```python
from build123d import *

# Parameters (mm, degrees)
BOSS_EXTRUDE1_DEPTH     = 12.7
FILLET2_SIZE            = 41.275
FILLET2_SIZE_2          = 69.85
FILLET3_R               = 25.4
FILLET4_R               = 19.05
FILLET6_R               = 127
CUT_EXTRUDE1_REACH      = 634.314
SKETCH3_W               = 241.600142069
SKETCH3_H               = 584.2
F_8_CLEARANCE_HOLE1_D   = 4.9149
F_1_4_CLEARANCE_HOLE1_D = 7.14248


with BuildPart() as part:
    # Sketch1 → Boss-Extrude1 (new body)
    with BuildSketch(Plane.XY):
        Polygon((-228.088766336, 0), (228.088766336, 0), (228.088766336, -443.878997916), (241.600142069, -584.2), (230.934597128, -584.2), (196.338766336, -463.55), (79.375, -463.55), (79.375, -363.22), (-79.375, -363.22), (-79.375, -463.55), (-196.338766336, -463.55), (-230.934597128, -584.2), (-241.600142069, -584.2), (-228.088766336, -443.878997916), align=None)
    extrude(amount=BOSS_EXTRUDE1_DEPTH)

    # Fillet2
    # a fillet whose section is not a circle: 69.85, 41.275 mm, written as the material it adds along each edge
    with BuildSketch(Plane(origin=(-79.375, -363.22, 0), x_dir=(1, 0, 0), z_dir=(0, 0, 1))) as fillet2_piece_1:
        with BuildLine():
            Bezier((FILLET2_SIZE, 0), (0, 0), (0, -FILLET2_SIZE_2), weights=[1, 1.5, 1])
            Line((0, -FILLET2_SIZE_2), (0, 0))
            Line((0, 0), (FILLET2_SIZE, 0))
        make_face()
    extrude(amount=12.7)

    # Fillet3
    fillet3_edges = [part.edges().sort_by_distance(p)[0] for p in [
        (-79.375, -463.55, 6.35),
    ]]
    fillet(fillet3_edges, radius=FILLET3_R)

    # Fillet4
    fillet4_edges = [part.edges().sort_by_distance(p)[0] for p in [
        (-196.338766336, -463.55, 6.35),
    ]]
    fillet(fillet4_edges, radius=FILLET4_R)

    # Fillet5
    # a fillet whose section is not a circle: 50.8, 22.225 mm, written as the material it takes off along each edge
    with BuildSketch(Plane(origin=(-230.934597128, -584.2, -116.185737858), x_dir=(0.2756373558169957, 0.9612616959383199, 0), z_dir=(0, 0, 1))) as fillet5_piece_1:
        with BuildLine():
            Bezier((46.474295143, 0), (0, 0), (-2.35779901, 8.222622324), weights=[1, 2.333333333, 1])
            Line((-2.35779901, 8.222622324), (0, 0))
            Line((0, 0), (46.474295143, 0))
        make_face()
    extrude(amount=245.071475716, mode=Mode.SUBTRACT)

    # Fillet6
    # the kernel refuses this fillet: 127 mm, written as the material it adds along each edge
    with BuildSketch(Plane(origin=(-228.088766336, -443.878997916, 0), x_dir=(0, 1, 0), z_dir=(0, 0, 1))) as fillet6_piece_1:
        with BuildLine():
            CenterArc((FILLET6_R * 0.0480334444852, FILLET6_R), FILLET6_R, 264.5, 5.5)
            Line((-FILLET6_R * 0.047812308035, FILLET6_R * 0.00460380163282), (0, 0))
            Line((0, 0), (FILLET6_R * 0.0480334444852, 0))
        make_face()
    extrude(amount=12.7)

    # Sketch3 → Cut-Extrude1 (cut, up to next)
    with BuildSketch(Plane.XY.offset(12.7), mode=Mode.PRIVATE) as cut_extrude1_sk1:
        with Locations((120.800071035, -292.1)):
            Rectangle(SKETCH3_W, SKETCH3_H)
    cut_extrude1_tool1 = extrude(cut_extrude1_sk1.sketch, amount=-CUT_EXTRUDE1_REACH, mode=Mode.PRIVATE) & part.part
    add(cut_extrude1_tool1.solids().sort_by_distance((120.800071, -292.1, 12.7))[0], mode=Mode.SUBTRACT)

    # Mirror5: part across plane


with BuildPart() as part_1:
    add(part.part)
    add(part.part.mirror(Plane(origin=(0, 0, -0.35025), x_dir=(0, 0, 1), z_dir=(-1, 0, 0))))

    # #8 Clearance Hole1 (through all)
    with Locations(Plane(origin=(0, 0, 0), x_dir=(-1, 0, 0), z_dir=(0, 0, -1))):
        with Locations((12.077216058, -342.5825), (-12.077216058, -342.5825)):
            Hole(F_8_CLEARANCE_HOLE1_D / 2)

    # 1/4 Clearance Hole1 (through all)
    with Locations(Plane(origin=(0, 0, 0), x_dir=(-1, 0, 0), z_dir=(0, 0, -1))):
        with Locations((0, -352.7425), (0, -332.4225)):
            Hole(F_1_4_CLEARANCE_HOLE1_D / 2)


solid = part_1.part
```
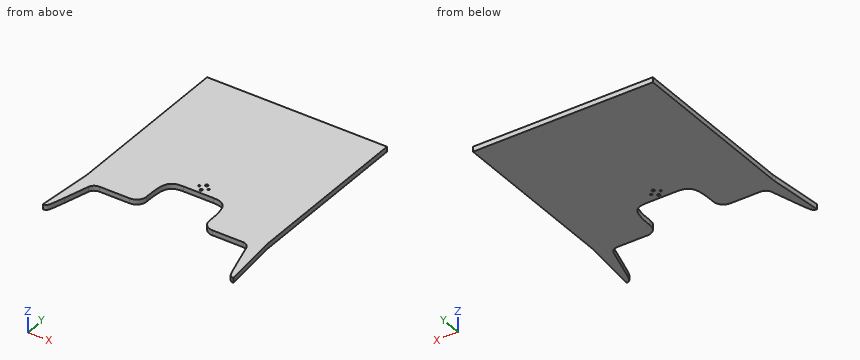
The listing builds one solid part. Answer for the finished solid, in the listing's coordinates (mm). Coordinates: 2 decimals unless noted, no trailing zeros. Loops run counter-clockwise (first coordinate to the right, second up) from the corner with the lowest first, then second, coordinate; pieces in that order, holes last. Notation, with made-up numbers: M 25,-6.5 L 71,-6.5 A36 cw 71,27.5 Z; hole C 61.5,50 d4. An arc over 180 degrees is marked long. Answer as CSV lines item,"result". Start each with the question number.
(1) The part is cut by section B-B (x = 127.5). Give the vertices of the cut face in (y, z).
(2) The part is cut by section A-A (y = -526). Give the vertices of the cut face in (x, z).
(3) The part is cut by section C-C (y = -93.5). Give the vertices of the cut face in (x, z), and give its area (3 significant figures).
(4) Given pin 1 (1.5 mm diameter, centred on y = -404, z = 8.5, fed in from +X); pin 2 (3 mm diameter, centred on y = -151, z = 7.5, fed in from -X); pin 3 (4 mm diameter, centred on x = 1.5, z = 5.5, fed in from -Y); pin 4 (3 mm diameter, centred on x = -12.08, y = -342.58, fed in from +Z), each flat-ended and moving along its own axis, determine where each tip first touches the part or whether it passes through.
(5) The part is cut by section D-D (z = 3.75). State how many separate pieces and enclosed holes the cut face has, and give its area (3 significant figures).
(6) Find the intervals of material crossed by L1, parallel to Y at x = 0, z = 9.5; L2, parallel to Y at x = -2, z = 2; L3, parallel to X at y = -343.5, z = 8, in increasing order. Write a range as [from, to].
Determined:
1,outline,"M -463.55,0 L 0,0 L 0,12.7 L -463.55,12.7 Z"
2,outline,"M -236,0 L -214.25,0 L -214.25,12.7 L -236,12.7 Z; M 214.25,0 L 236,0 L 236,12.7 L 214.25,12.7 Z"
3,outline,"M -228.09,0 L 228.09,0 L 228.09,12.7 L -228.09,12.7 Z"
3,area,"5,790 mm2"
4,pin 1,"x = 228.09"
4,pin 2,"x = -228.09"
4,pin 3,"y = -363.22"
4,pin 4,"through"
5,separate pieces,"1"
5,enclosed holes,"4"
5,area,"201,000 mm2"
6,L1,"[-363.22, -356.31], [-349.17, -335.99], [-328.85, 0]"
6,L2,"[-363.22, -355.7], [-349.78, -335.38], [-329.46, 0]"
6,L3,"[-228.09, -14.36], [-9.8, 9.8], [14.36, 228.09]"
